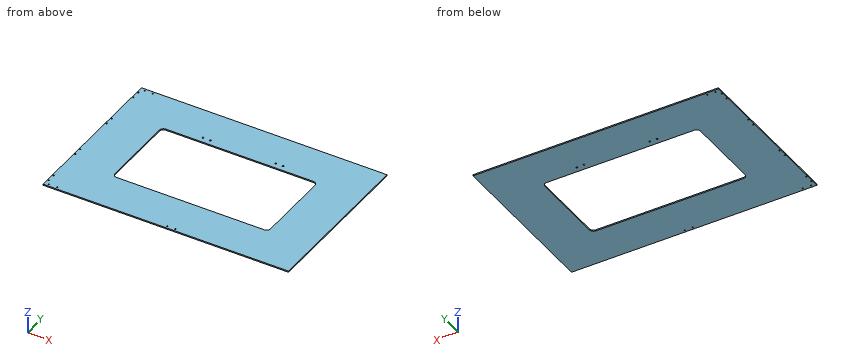
from build123d import *

# Parameters (mm, degrees)
SKETCH_1_W          = 600
SKETCH_1_H          = 400
EXTRUDE_1_DEPTH     = 3
SKETCH_2_R          = 1.6
CUT_EXTRUDE_1_DEPTH = 361.567608085
SKETCH_4_R          = 1.6
CUT_EXTRUDE_2_DEPTH = 361.567608085
SKETCH_6_R          = 1.6
CUT_EXTRUDE_3_DEPTH = 361.567608085
SKETCH_7_W          = 380.5
SKETCH_7_H          = 200.5
CUT_EXTRUDE_4_DEPTH = 361.567608085
SKETCH_8_R          = 1.575
CUT_EXTRUDE_5_DEPTH = 361.567608085
SKETCH_9_R          = 2
CUT_EXTRUDE_6_DEPTH = 361.567608085
FILLET_1_R          = 10


with BuildPart() as part:
    # 草图1 → 凸台-拉伸1 (new body)
    with BuildSketch(Plane.XY):
        Rectangle(SKETCH_1_W, SKETCH_1_H)
    extrude(amount=EXTRUDE_1_DEPTH)

    # 草图2 → 切除-拉伸1 (cut, through all)
    with BuildSketch(Plane.XY.offset(3)):
        with Locations((-297, 162)):
            Circle(SKETCH_2_R)
        with Locations((-297, 182)):
            Circle(SKETCH_2_R)
        with Locations((-289, 194)):
            Circle(SKETCH_2_R)
        with Locations((-269, 194)):
            Circle(SKETCH_2_R)
    extrude(amount=-CUT_EXTRUDE_1_DEPTH, mode=Mode.SUBTRACT)

    # 草图4 → 切除-拉伸2 (cut, through all)
    with BuildSketch(Plane.XY.offset(3)):
        with Locations((-297, -162)):
            Circle(SKETCH_4_R)
        with Locations((-297, -182)):
            Circle(SKETCH_4_R)
        with Locations((-289, -194)):
            Circle(SKETCH_4_R)
        with Locations((-269, -194)):
            Circle(SKETCH_4_R)
    extrude(amount=-CUT_EXTRUDE_2_DEPTH, mode=Mode.SUBTRACT)

    # 草图6 → 切除-拉伸3 (cut, through all)
    with BuildSketch(Plane(origin=(0, 0, 0), x_dir=(-1, 0, 0), z_dir=(0, 0, -1))):
        with Locations((0, -194)):
            Circle(SKETCH_6_R)
        with Locations((-20, -194)):
            Circle(SKETCH_6_R)
    extrude(amount=-CUT_EXTRUDE_3_DEPTH, mode=Mode.SUBTRACT)

    # 草图7 → 切除-拉伸4 (cut, through all)
    with BuildSketch(Plane.XY.offset(3)):
        Rectangle(SKETCH_7_W, SKETCH_7_H)
    extrude(amount=-CUT_EXTRUDE_4_DEPTH, mode=Mode.SUBTRACT)

    # 草图8 → 切除-拉伸5 (cut, through all)
    with BuildSketch(Plane.XY.offset(3)):
        with Locations((-297, 73.5)):
            Circle(SKETCH_8_R)
        with Locations((-297, 53.5)):
            Circle(SKETCH_8_R)
        with Locations((-297, -53.5)):
            Circle(SKETCH_8_R)
        with Locations((-297, -73.5)):
            Circle(SKETCH_8_R)
    extrude(amount=-CUT_EXTRUDE_5_DEPTH, mode=Mode.SUBTRACT)

    # 草图9 → 切除-拉伸6 (cut, through all)
    with BuildSketch(Plane.XY.offset(3)):
        with Locations((-98, 114)):
            Circle(SKETCH_9_R)
        with Locations((-80, 114)):
            Circle(SKETCH_9_R)
        with Locations(Location((80, 114, 0), (0, 0, 180))):
            Circle(SKETCH_9_R)
        with Locations(Location((98, 114, 0), (0, 0, 180))):
            Circle(SKETCH_9_R)
    extrude(amount=-CUT_EXTRUDE_6_DEPTH, mode=Mode.SUBTRACT)

    # 圆角1
    fillet_1_edges = [part.edges().sort_by_distance(p)[0] for p in [
        (190.25, 100.25, 1.5),
        (190.25, -100.25, 1.5),
        (-190.25, -100.25, 1.5),
        (-190.25, 100.25, 1.5),
    ]]
    fillet(fillet_1_edges, radius=FILLET_1_R)


solid = part.part
Can you work these out from the model? Positions are in its coordinate system, mm. Give positions to 0.01 mm unless a question says otherwise; leave off trailing zeros. Order: outer loops, then holes, each group sorted by start corner. A loop starts at its lowest first (then second) coordinate and runs counter-clockwise, first axis right, second up. Notation, with made-up numbers: M 28,-39 L 61,-39 A20 cw 61,-7 Z; hole C 71.5,57 d7. An arc over 180 degrees is marked long. One line per item, written item: value.
Item 1: If we section it at B-B on x = 166: Write out the boundary of the cut face in (y, z), and give its area (4 significant figures).
Verdict:
outline: M -200,0 L -100.25,0 L -100.25,3 L -200,3 Z; M 100.25,0 L 200,0 L 200,3 L 100.25,3 Z
area: 598.5 mm2
Item 2: For pin 1 (4 mm diameter, centred on x = 20, y = -194, fed in from -Z), with a flat end and sliding along its axis, tell me the tip position at first contact or that it passes through.
Verdict:
pin 1: z = 0
Item 3: Please list where these lines run through material, in increasing order: line 1 (Y direction, x = 0, z = 2.3); line 2 (X direction, y = -194, z = 1.95); line 3 (X direction, y = 194, z = 2.25).
Verdict:
line 1: -200 to -195.6, -192.4 to -100.25, 100.25 to 200
line 2: -300 to -290.6, -287.4 to -270.6, -267.4 to -1.6, 1.6 to 18.4, 21.6 to 300
line 3: -300 to -290.6, -287.4 to -270.6, -267.4 to 300
Item 4: If we section it at A-A on z = 1.9: State how many separate pieces and enclosed holes the cut face has, and give its area (3 significant figures).
Verdict:
separate pieces: 1
enclosed holes: 19
area: 164,000 mm2
Item 5: If we section it at C-C on y = -64: Write out the boundary of the cut face in (x, z).
Verdict:
outline: M -300,0 L -190.25,0 L -190.25,3 L -300,3 Z; M 190.25,0 L 300,0 L 300,3 L 190.25,3 Z
